Input: part model. Units: mm. Frame: model coordinates. A direction names the side the tool comes from. Give positions to 0.01 mm unless a question says otherwise; leave off trailing zeros. Loops run counter-clockwise (first coordinate to the right, second up) from the corner with the lowest first, then second, coordinate; pieces in that order, holes last. Notation, with made-up numbers: M 46.25,-18.75 L 54.25,-18.75 A15 cw 54.25,-2.75 Z; hole C 17.5,18.5 d4. An arc over 180 degrees is marked long. Use CSV: the item, a comma, the result in double quotes. Start each with the question number.
Q1. Pull-direction query (Y, two-part tool) for faces 4 (the cylindrical face through (-5.157, 19.79, 1.479)), 5 (the cylindrical face through (-22.27, 43.85, 1.48)), 6 (the cylindrical face through (-3.094, 19.537, 1.479)); classes: released by +Y, released by -Y, zero draft, split by the parting line, or undercut.
Q2. Section D-D, the plane y = 14. Output: boundary loops of the cut face in (x, z).
Q3. Pin query (flat end, axial travel): pin 1 (5 mm diameter, centred on x = -19.27, y = 43.77, fed in from -Z). Return the tip coordinate at first contact, or that it passes through.
Q4. Section B-B, the plane y = 28. Output: boundary loops of the cut face in (x, z).
Q5. Section A-A, the plane x = 0. Output: boundary loops of the cut face in (y, z).
Q6. Section C-C, the plane x = -11.5. Output: boundary loops of the cut face in (y, z).
Q7. Reachability of faces 1 (the cylindrical face through (-0.82, 15.7, 1.48)), 2 (the cylindrical face through (-4.04, 32.76, 1.48)), 3 (the cylindrical face through (1.13, 9.29, 1.48)) from +Z, -Z, +X, -X, +Y, -Y: full face, straight path, thin tool, end or side. Return the list, or none.
Q8. Material intervals for line 1 along Y through (x, z) = (0, 1.35); line 2 along X through (y, z) = (0.5, 1.2); line 3 along Y through (x, z) = (1.25, 1.75), sorted ascending.
from build123d import *

# Parameters (mm, degrees)
BOSS_EXTRUDE1_OUTLINE_R = 1.5
BOSS_EXTRUDE1_DEPTH     = 3
FILLET1_R               = 5
CUT_EXTRUDE1_DEPTH      = 3


# Read off the part's stored shape, not the designer's step: Boss-Extrude1
with BuildPart() as part:
    # Boss-Extrude1 outline → Boss-Extrude1 (new body)
    with BuildSketch(Plane.XY):
        with BuildLine():
            ThreePointArc((-9.577975431, 41.29578544), (-7.088317742, 38.60475873), (-5.596455347, 35.255972867))
            add(Edge.make_bspline(
                [(-5.596455347, 35.255972867), (-5.582747417, 35.202444502), (-5.55529889, 35.095260217), (-5.517467472, 34.934551052), (-5.482131356, 34.775084793), (-5.449615345, 34.617937051), (-5.419947602, 34.464275495), (-5.393218029, 34.315238656), (-5.368054814, 34.162831666), (-5.344795736, 34.008181607), (-5.322858552, 33.847412998), (-5.30329297, 33.684837729), (-5.293582635, 33.591977311), (-5.288408722, 33.542498925)],
                knots=[0, 0, 0, 0, 0.07878117, 0.157750071, 0.236927243, 0.316333061, 0.395987726, 0.475911251, 0.556123446, 0.652047242, 0.7511991, 0.867432569, 1, 1, 1, 1], degree=3))
            Line((-5.288408722, 33.542498925), (-6.480466419, 33.453304935))
            Line((-6.480466419, 33.453304935), (-5.341603358, 18.232655185))
            Line((-5.341603358, 18.232655185), (-4.147731483, 18.321984917))
            ThreePointArc((-4.147731483, 18.321984917), (-4.032924942, 17.489163116), (-3.846988472, 16.66928488))
            ThreePointArc((-3.846988472, 16.66928488), (-2.642137665, 13.858181692), (-0.627607898, 11.55695671))
            ThreePointArc((-0.627607898, 11.55695671), (1.144975693, 9.256897759), (1.771644479, 6.421477156))
            ThreePointArc((1.771644479, 6.421477156), (1.098096567, 4.533436187), (-0.614174692, 3.491086617))
            ThreePointArc((-0.614174692, 3.491086617), (-1.806361188, -1.840587951), (2.992161355, 0.771354572))
            ThreePointArc((2.992161355, 0.771354572), (3.041722898, 1.572124284), (3.301741951, 2.331122684))
            ThreePointArc((3.301741951, 2.331122684), (4.077870779, 8.309876297), (0.972698011, 13.47763914))
            ThreePointArc((0.972698011, 13.47763914), (-0.835685645, 15.731138378), (-1.624382222, 18.510790869))
            Line((-1.624382222, 18.510790869), (-0.35554127, 18.605730055))
            Line((-0.35554127, 18.605730055), (-1.494404331, 33.826379806))
            Line((-1.494404331, 33.826379806), (-2.713176612, 33.735186936))
            add(Edge.make_bspline(
                [(-2.713176612, 33.735186936), (-2.713923066, 33.740199809), (-2.719747517, 33.779179521), (-2.737276775, 33.893529306), (-2.771774985, 34.097834296), (-2.823249297, 34.37037297), (-2.883340819, 34.657944683), (-2.950356176, 34.952197534), (-3.001326008, 35.14925666), (-3.026538809, 35.246734176)],
                knots=[0.162262456, 0.162262456, 0.162262456, 0.162262456, 0.173543134, 0.249389735, 0.406042985, 0.559353198, 0.709395257, 0.856249091, 1, 1, 1, 1], degree=3))
            ThreePointArc((-3.026538809, 35.246734176), (-4.904423993, 39.832081027), (-8.286103826, 43.453696691))
            ThreePointArc((-8.286103826, 43.453696691), (-9.376853546, 46.101850718), (-12.192055187, 46.62824831))
            ThreePointArc((-12.192055187, 46.62824831), (-15.268978264, 46.143107446), (-18.345901341, 46.62824831))
            ThreePointArc((-18.345901341, 46.62824831), (-22.268978264, 43.77379057), (-18.345901341, 40.919332829))
            ThreePointArc((-18.345901341, 40.919332829), (-15.268978264, 41.404473693), (-12.192055187, 40.919332829))
            ThreePointArc((-12.192055187, 40.919332829), (-10.841360803, 40.804423077), (-9.577975431, 41.29578544))
        make_face()
        with Locations((0, 0.55462796)):
            Circle(BOSS_EXTRUDE1_OUTLINE_R, mode=Mode.SUBTRACT)
        with Locations((-19.268978264, 43.773790569)):
            Circle(BOSS_EXTRUDE1_OUTLINE_R, mode=Mode.SUBTRACT)
        with Locations((-11.268978264, 43.773790569)):
            Circle(BOSS_EXTRUDE1_OUTLINE_R, mode=Mode.SUBTRACT)
    extrude(amount=BOSS_EXTRUDE1_DEPTH)

    # Fillet1
    # the kernel refuses this fillet: 5 mm, written as the material it takes off along each edge
    with BuildSketch(Plane(origin=(-6.480466419, 33.453304935, -8.110541878), x_dir=(0.9972124174989766, 0.07461497427357966, 0), z_dir=(0, 0, 1))) as fillet1_piece_1:
        with BuildLine():
            CenterArc((4.999999999, -3.244216752), FILLET1_R, 139.545547884, 40.454452104)
            Line((-1e-09, -3.244216751), (-0.100000001, -3.244216751))
            Line((-0.100000001, -3.244216751), (-0.1, 0))
            Line((-0.1, 0), (0, 0.1))
            ThreePointArc((0, 0.1), (0.597694973, 0.1), (1.119297744, 0.064884335))
            Line((1.119297744, 0.064884335), (1.195389945, 0))
        make_face()
    extrude(amount=19.221083756, mode=Mode.SUBTRACT)
    with BuildSketch(Plane(origin=(-1.494404331, 33.826379806, -8.188433173), x_dir=(0.07461497405549736, -0.9972124175152941, 0), z_dir=(0, 0, 1))) as fillet1_piece_2:
        with BuildLine():
            CenterArc((3.275373269, -5), FILLET1_R, 90, 40.925310843)
            Line((0, -1.222179206), (-0.065507465, -1.14662279))
            ThreePointArc((-0.065507465, -1.14662279), (-0.1, -0.611089603), (-0.1, 0))
            Line((-0.1, 0), (0, 0.1))
            Line((0, 0.1), (3.275373269, 0.1))
            Line((3.275373269, 0.1), (3.275373269, 0))
        make_face()
    extrude(amount=19.376866346, mode=Mode.SUBTRACT)
    with BuildSketch(Plane(origin=(-5.341603358, 18.232655185, -8.115872597), x_dir=(-0.07461497406037235, 0.9972124175149295, 0), z_dir=(0, 0, 1))) as fillet1_piece_3:
        with BuildLine():
            CenterArc((3.246349039, -5), FILLET1_R, 90, 40.486571122)
            Line((-1e-09, -1.197209194), (-0.064926982, -1.121153378))
            ThreePointArc((-0.064926982, -1.121153378), (-0.1, -0.598604597), (-0.1, 0))
            Line((-0.1, 0), (0, 0.1))
            Line((0, 0.1), (3.246349039, 0.1))
            Line((3.246349039, 0.1), (3.246349039, 0))
        make_face()
    extrude(amount=19.231745194, mode=Mode.SUBTRACT)
    with BuildSketch(Plane(origin=(-0.35554127, 18.605730055, -8.33100668), x_dir=(-0.9972124174875004, -0.07461497442695494, 0), z_dir=(0, 0, 1))) as fillet1_piece_4:
        with BuildLine():
            CenterArc((4.999999999, -3.332402674), FILLET1_R, 138.203991534, 41.796008444)
            Line((-1e-09, -3.332402672), (-0.100000001, -3.332402672))
            Line((-0.100000001, -3.332402672), (-0.1, 0))
            Line((-0.1, 0), (0, 0.1))
            ThreePointArc((0, 0.1), (0.636193919, 0.1), (1.197835595, 0.066648053))
            Line((1.197835595, 0.066648053), (1.272387838, 0))
        make_face()
    extrude(amount=19.662013359, mode=Mode.SUBTRACT)

    # Sketch2 → Cut-Extrude1 (cut)
    with BuildSketch(Plane(origin=(0, 0, 0), x_dir=(-1, 0, 0), z_dir=(0, 0, -1))):
        with BuildLine():
            Line((5.006415896, 31.658546167), (4.17027649, 20.483730275))
            ThreePointArc((4.17027649, 20.483730275), (3.071829301, 19.538219294), (2.12631832, 20.636666483))
            Line((2.12631832, 20.636666483), (2.962457726, 31.811482375))
            ThreePointArc((2.962457726, 31.811482375), (4.060904915, 32.756993356), (5.006415896, 31.658546167))
        make_face()
    extrude(amount=-CUT_EXTRUDE1_DEPTH, mode=Mode.SUBTRACT)


solid = part.part
A:
1,face 4,"released by -Y"
1,face 5,"split by the parting line"
1,face 6,"undercut"
2,outline,"M -2.73,0 L 0.41,0 L 0.41,3 L -2.73,3 Z"
3,pin 1,"z = 0"
4,outline,"M -6.07,0 L -4.73,0 L -4.73,3 L -6.07,3 Z; M -2.68,0 L -1.06,0 L -1.06,3 L -2.68,3 Z"
5,outline,"M -2.45,0 L -0.95,0 L -0.95,3 L -2.45,3 Z; M 2.05,0 L 3.69,0 L 3.69,3 L 2.05,3 Z; M 10.96,0 L 14.46,0 L 14.46,3 L 10.96,3 Z"
6,outline,"M 40.78,0 L 42.29,0 L 42.29,3 L 40.78,3 Z; M 45.26,0 L 46.76,0 L 46.76,3 L 45.26,3 Z"
7,face 1,"+Z, -Z, +X"
7,face 2,"+Z, -Z"
7,face 3,"+Z, -Z, -X"
8,line 1,"-2.45 to -0.95, 2.05 to 3.69, 10.96 to 14.46"
8,line 2,"-3 to -1.5, 1.5 to 3"
8,line 3,"-2.17 to -0.27, 1.38 to 4.74, 9.02 to 13.24"
